```python
from build123d import *

# Parameters (mm, degrees)
SKETCH1_R               = 0.375
BOSS_EXTRUDE1_DEPTH     = 20.25
SKETCH3_R               = 0.25
CUT_EXTRUDE1_DEPTH      = 6.5
SKETCH4_R               = 0.25
CUT_EXTRUDE2_DEPTH      = 6.5
SKETCH5_W               = 0.3
SKETCH5_H               = 0.1
CUT_EXTRUDE3_DEPTH      = 1.25
SKETCH6_W               = 0.5
SKETCH6_H               = 0.1
CUT_EXTRUDE4_DEPTH      = 1.25
SKETCH7_W               = 5.25772593
SKETCH7_H               = 0.43012496
CUT_EXTRUDE5_DEPTH      = 1.375
CUT_EXTRUDE5_DEPTH_BACK = 1.375
BOSS_EXTRUDE2_DEPTH     = 0.375
LPATTERN1_COUNT         = 12
LPATTERN1_PITCH         = 0.4


with BuildPart() as part:
    # Sketch1 → Boss-Extrude1 (new body)
    with BuildSketch(Plane(origin=(0, 0, 0), x_dir=(0, 0, -1), z_dir=(1, 0, 0))):
        Circle(SKETCH1_R)
    extrude(amount=BOSS_EXTRUDE1_DEPTH)

    # Sketch3 → Cut-Extrude1 (cut)
    with BuildSketch(Plane(origin=(0, 0, 0), x_dir=(0, 0, -1), z_dir=(1, 0, 0))):
        Circle(SKETCH3_R)
    extrude(amount=CUT_EXTRUDE1_DEPTH, mode=Mode.SUBTRACT)

    # Sketch4 → Cut-Extrude2 (cut)
    with BuildSketch(Plane(origin=(20.25, 0, 0), x_dir=(0, 0, -1), z_dir=(1, 0, 0))):
        Circle(SKETCH4_R)
    extrude(amount=-CUT_EXTRUDE2_DEPTH, mode=Mode.SUBTRACT)

    # Sketch5 → Cut-Extrude3 (cut)
    with BuildSketch(Plane(origin=(20.25, 0, 0), x_dir=(0, 0, -1), z_dir=(1, 0, 0))):
        with Locations((0, 0.371911734)):
            Rectangle(SKETCH5_W, SKETCH5_H)
    extrude(amount=-CUT_EXTRUDE3_DEPTH, mode=Mode.SUBTRACT)

    # Sketch6 → Cut-Extrude4 (cut)
    with BuildSketch(Plane(origin=(0, 0, 0), x_dir=(0, 0, -1), z_dir=(1, 0, 0))):
        with Locations((0, 0.375)):
            Rectangle(SKETCH6_W, SKETCH6_H)
    extrude(amount=CUT_EXTRUDE4_DEPTH, mode=Mode.SUBTRACT)

    # Sketch7 → Cut-Extrude5 (cut, two sides)
    with BuildSketch(Plane.XY) as cut_extrude5_sk:
        with Locations((10.125, 0.21506248)):
            Rectangle(SKETCH7_W, SKETCH7_H)
    extrude(amount=CUT_EXTRUDE5_DEPTH, mode=Mode.SUBTRACT)
    extrude(cut_extrude5_sk.sketch, amount=-CUT_EXTRUDE5_DEPTH_BACK, mode=Mode.SUBTRACT)

    # Sketch8 → Boss-Extrude2 (add, symmetric)
    with BuildSketch(Plane.XY):
        Polygon((7.746137035, 0), (7.875912836, 0.356556082), (7.925912836, 0.356556082), (8.055688636, 0), align=None)
    boss_extrude2 = extrude(amount=BOSS_EXTRUDE2_DEPTH, both=True)

    # LPattern1: Boss-Extrude2 ×12
    with Locations(*[(i * LPATTERN1_PITCH, 0, 0) for i in range(1, LPATTERN1_COUNT)]):
        add(boss_extrude2)


solid = part.part
```
Build history of the part. All positions in model axes, mm. Coordinates: 2 decimals unless noted, no trailing zeros. Order: outer loops, then holes, each group sorted by start corner. A loop starts at its lowest first (then second) coordinate and runs counter-clockwise, first axis right, second up.
Item 1: Saw through at B-B on x = 13. List the corners of the cut face in (y, z) (3 decimals).
Filled in:
outline: circle Ø0.75 at (0, 0)
Item 2: Drill centre lines: L1, parallel to X at y = -0.2, z = 0; L2, parallel to Z at x = 11, y = -0.05; L3, parallel to Y at x = 13.5, z = -0.2. Where is each one in solid material? Low to high.
Filled in:
L1: x = 6.5 to 13.75
L2: z = -0.37 to 0.37
L3: y = -0.32 to 0.32
Item 3: Saw through at A-A on x = 2. List the corners of the cut face in (y, z) (3 decimals), then the cut area to 3 significant figures.
Filled in:
outline: circle Ø0.75 at (0, 0); hole circle Ø0.5 at (0, 0)
area: 0.245 mm2
